Here's how the part is built. I have some questions about the finished solid (model axes, mm). A direction names the side the tool comes from. Round coordinates to 2 decimals unless told otherwise and drop trailing zeros. Loops run counter-clockwise (first coordinate to the right, second up) from the corner with the lowest first, then second, coordinate; pieces in that order, holes last. Notation, with made-up numbers: (16.25, 17.25) -> (48.25, 17.25) arc R27 ccw to (48.25, 48.25) -> close; hole circle Ø9 at (55, 1.5). An arc over 180 degrees is marked (long way). Use one line per item in the form item = value. Start each with the question number.
Item 1: If we section it at B-B (z = 1.2): Write out the boundary of the cut face in (x, y), then the cut area to 3 significant figures.
Item 2: If we section it at C-C (x = -1.5): Write out the boundary of the cut face in (y, z), then the cut area to 3 significant figures.
Item 3: If we section it at A-A (y = 0): Write out the boundary of the cut face in (x, z), then the cut area to 3 significant figures.
Item 4: If we section it at D-D (y = 22): Write out the boundary of the cut face in (x, z).
Item 5: For faces 1 (the face through (3.75, 19, 3)), 2 (the face through (-1.5, 2.6, 3)), 3 (the face through (-3.75, 19, 3)), which set-ups out of +Z, -Z, +X, -X, +Y, -Y let a thin tool reach every point of the face, with its end or its side?
Item 6: Thinking about a two-plate mould opening in X: for faces 4 (the face through (4.425, 8.712, 2.958)), 5 (the face through (0, 6, 6)), 6 (the face through (1.5, -2.6, 3)), which applies, released by +X, released by -X, zero draft, split by the parting line, or undercut?
Item 7: If I drill on L1, parallel to X at y = 0, z = 3.55; L2, parallel to Y at x = -0.25, z = 4.2; L3, parallel to Y at x = 0.5, z = 1.2, over which ranges is the centre line in solid material (lowest first)? Write a range as [from, to].
Item 8: I'm going to push flat-ended pins straight in: pin 1 Ø3 at (y, z) = (21.5, 2.5) entering from -X; pin 2 Ø3 at (y, z) = (9, 2.5) entering from -X; pin 3 Ø3 at (y, z) = (9.5, 3) entering from -X. Where does each tip first touch, or does it pass through?
```python
from build123d import *

# Parameters (mm, degrees)
BOSS_EXTRUDE1_DEPTH = 6


with BuildPart() as part:
    # Sketch1 → Boss-Extrude1 (new body)
    with BuildSketch(Plane.XY):
        with BuildLine():
            Line((-3.75, 13.863170633), (-3.75, 23.75))
            ThreePointArc((-3.75, 23.75), (0, 27.5), (3.75, 23.75))
            Line((3.75, 23.75), (3.75, 13.863170633))
            ThreePointArc((3.75, 13.863170633), (4.443854017, 8.640840954), (6.477272727, 3.780864718))
            ThreePointArc((6.477272727, 3.780864718), (0, -7.5), (-6.477272727, 3.780864718))
            ThreePointArc((-6.477272727, 3.780864718), (-4.443854017, 8.640840954), (-3.75, 13.863170633))
        make_face()
        Polygon((0, 3.464101615), (-3, 1.732050808), (-3, -1.732050808), (0, -3.464101615), (3, -1.732050808), (3, 1.732050808), align=None, mode=Mode.SUBTRACT)
    extrude(amount=BOSS_EXTRUDE1_DEPTH)


solid = part.part
```
Values found:
q1.outline = (-6.48, 3.78) arc R7.5 ccw (long way) to (6.48, 3.78) arc R20 cw to (3.75, 13.86) -> (3.75, 23.75) arc R3.75 ccw to (-3.75, 23.75) -> (-3.75, 13.86) arc R20 cw to start; hole (-3, -1.73) -> (0, -3.46) -> (3, -1.73) -> (3, 1.73) -> (0, 3.46) -> (-3, 1.73) -> close
q1.area = 301 mm2
q2.outline = (-7.35, 0) -> (-2.6, 0) -> (-2.6, 6) -> (-7.35, 6) -> close; (2.6, 0) -> (27.19, 0) -> (27.19, 6) -> (2.6, 6) -> close
q2.area = 176 mm2
q3.outline = (-7.5, 0) -> (-3, 0) -> (-3, 6) -> (-7.5, 6) -> close; (3, 0) -> (7.5, 0) -> (7.5, 6) -> (3, 6) -> close
q3.area = 54.0 mm2
q4.outline = (-3.75, 0) -> (3.75, 0) -> (3.75, 6) -> (-3.75, 6) -> close
q5.face_1 = +Z, -Z, +X, +Y
q5.face_2 = +Z, -Z
q5.face_3 = +Z, -Z, -X, +Y
q6.face_4 = released by +X
q6.face_5 = zero draft
q6.face_6 = undercut
q7.L1 = [-7.5, -3], [3, 7.5]
q7.L2 = [-7.5, -3.32], [3.32, 27.49]
q7.L3 = [-7.48, -3.18], [3.18, 27.47]
q8.pin_1 = -3.75
q8.pin_2 = -4.79
q8.pin_3 = -4.63
